```python
from build123d import *

# Parameters (mm, degrees)
SKETCH1_W           = 14
SKETCH1_H           = 3
BOSS_EXTRUDE1_DEPTH = 16
BOSS_EXTRUDE2_DEPTH = 2
SKETCH3_R           = 3.41
CUT_EXTRUDE2_DEPTH  = 7.8


with BuildPart() as part:
    # Sketch1 → Boss-Extrude1 (new body)
    with BuildSketch(Plane.XY):
        Rectangle(SKETCH1_W, SKETCH1_H)
    extrude(amount=BOSS_EXTRUDE1_DEPTH)

    # Sketch2 → Boss-Extrude2 (add)
    with BuildSketch(Plane.XY.offset(16)):
        with BuildLine():
            Line((-7, 1.5), (7, 1.5))
            ThreePointArc((7, 1.5), (5.80980001, 5.404641321), (2.643936044, 7.981481481))
            ThreePointArc((2.643936044, 7.981481481), (0, 18.30430246), (-2.643936044, 7.981481481))
            ThreePointArc((-2.643936044, 7.981481481), (-5.80980001, 5.404641321), (-7, 1.5))
        make_face()
    boss_extrude2 = extrude(amount=-BOSS_EXTRUDE2_DEPTH)

    # Sketch3 → Cut-Extrude2 (cut)
    with BuildSketch(Plane.XY.offset(16)):
        with Locations((0, 12.80430246)):
            Circle(SKETCH3_R)
    cut_extrude2 = extrude(amount=-CUT_EXTRUDE2_DEPTH, mode=Mode.SUBTRACT)

    # Mirror1: Boss-Extrude2, Cut-Extrude2 across plane
    add(boss_extrude2.mirror(Plane(origin=(0, 0, 8), x_dir=(1, 0, 0), z_dir=(0, 0, -1))))
    add(cut_extrude2.mirror(Plane(origin=(0, 0, 8), x_dir=(1, 0, 0), z_dir=(0, 0, -1))), mode=Mode.SUBTRACT)


solid = part.part
```
The model under review builds one solid part; all positions refer to its coordinate system, in mm. A direction names the side the tool comes from. Give positions to 0.01 mm unless a question says otherwise; leave off trailing zeros. Loops run counter-clockwise (first coordinate to the right, second up) from the corner with the lowest first, then second, coordinate; pieces in that order, holes last. Notation, with made-up numbers: (-3.5, -11.5) -> (18.5, -11.5) arc R19 ccw to (18.5, 8.5) -> close; hole circle Ø5 at (-8, 79). An arc over 180 degrees is marked (long way). Use CSV: the item, a comma, the result in double quotes.
1. Consider section B-B, the plane y = 9. Write out the cut boundary in (x, z), then the cut area to 3 significant figures.
Result:
outline,"(-3.97, 0) -> (3.97, 0) -> (3.97, 2) -> (-3.97, 2) -> close; (-3.97, 14) -> (3.97, 14) -> (3.97, 16) -> (-3.97, 16) -> close"
area,"31.8 mm²"
2. Machinability: for faces 1 (the face through (0, 6, 0)), 2 (the face through (0, 1.5, 8)), which of the approach directions +Z, -Z, +X, -X, +Y, -Y give a long, thin tool a straight path to every point of the face, cutting with its end or side? Answer none if there is none.
Result:
face 1,"-Z, +X, -X, +Y, -Y"
face 2,"+X, -X, +Y"
3. Consider section A-A, the plane x = 0. Write out the cut boundary in (y, z).
Result:
outline,"(-1.5, 0) -> (9.39, 0) -> (9.39, 2) -> (1.5, 2) -> (1.5, 14) -> (9.39, 14) -> (9.39, 16) -> (-1.5, 16) -> close; (16.21, 0) -> (18.3, 0) -> (18.3, 2) -> (16.21, 2) -> close; (16.21, 14) -> (18.3, 14) -> (18.3, 16) -> (16.21, 16) -> close"
4. To check wall thickness, follow probe 1 along Y at (x, z) = (0, 0.7); probe 2 along Z at (x, y) = (0.5, 3.25); probe 3 along X at (y, z) = (13, 15.75). State the ranges of each line that lie inside material, in increasing order. Write a range as from..to.
Result:
probe 1,"y = -1.5..9.39, 16.21..18.3"
probe 2,"z = 0..2, 14..16"
probe 3,"x = -5.5..-3.4, 3.4..5.5"
5. For P1, Ø5, axis at x = 5.5, z = 7.5, coming from the +Y side; P2, Ø7, axis at x = 2, y = 13, coming from the -Z side; P3, Ø2, axis at x = 5, z = 2.5, coming from the +Y side; P4, Ø3, axis at y = 4, z = 10.5, coming from the +X side, all flat-tipped, find the tip position at first contact; note any pin that passes through.
Result:
P1,"stops at y = 1.5"
P2,"stops at z = 0"
P3,"stops at y = 16.43"
P4,"passes through"
6. The part is to be moulded in two halves that separate along Z. For faces 3 (the face through (0, 8, 2)), 4 (the face through (0, 6, 16)), 5 (the face through (0, -1.5, 8)), say which applies: +Z half, -Z half, draft (parallel to the pull), parting line (faces both ways), or undercut.
Result:
face 3,"undercut"
face 4,"+Z half"
face 5,"draft"
7. Consider section D-D, the plane y = 14. Write out the cut boundary in (x, z), then the cut area to 3 significant figures.
Result:
outline,"(-5.37, 0) -> (-3.19, 0) -> (-3.19, 2) -> (-5.37, 2) -> close; (-5.37, 14) -> (-3.19, 14) -> (-3.19, 16) -> (-5.37, 16) -> close; (3.19, 0) -> (5.37, 0) -> (5.37, 2) -> (3.19, 2) -> close; (3.19, 14) -> (5.37, 14) -> (5.37, 16) -> (3.19, 16) -> close"
area,"17.4 mm²"
8. Consider section C-C, the plane z = 14.5. Write out the cut boundary in (x, y).
Result:
outline,"(-7, -1.5) -> (7, -1.5) -> (7, 1.5) arc R7 ccw to (2.64, 7.98) arc R5.5 ccw (long way) to (-2.64, 7.98) arc R7 ccw to (-7, 1.5) -> close; hole circle Ø6.82 at (0, 12.8)"
